Build history of the part. All positions in model axes, mm. A direction names the side the tool comes from. Round coordinates to 2 decimals unless told otherwise and drop trailing zeros. Order: outer loops, then holes, each group sorted by start corner. A loop starts at its lowest first (then second) coordinate and runs counter-clockwise, first axis right, second up. Notation, with made-up numbers: (-34.5, 56) -> (22.5, 56) arc R27 ccw to (22.5, 76) -> close; hole circle Ø3 at (-38.5, -16). An arc over 180 degrees is marked (long way). Use a Markdown table: item, result. Add a question column.
Item 1: 3-axis set-ups, long thin cutter, end or side, ignore diameter. For faces 1 (the face through (-25.126, -37, 2)), 2 (the face through (-9.126, 36, 6)), 3 (the face through (-15.126, -43, 6)): which of +Z, -Z, +X, -X, +Y, -Y reach the whole face in a straight line?
Item 2: Slice it at A-A, the plane y = -38.5. Give the cut face in (x, z), plus the area to 3 significant figures.
Item 3: Pin check, flat tips, straight feed: pin 1 (3 mm diameter, centred on y = -10.5, z = 3, fed in from -X); pin 2 (2 mm diameter, centred on y = 29.5, z = 2.5, fed in from +X); pin 3 (2.5 mm diameter, centred on x = 8.5, z = 6, fed in from +Y). Stop position of each tip, or through.
Item 4: Probe L1, parallel to X at y = -49, z = 5.25; L2, parallel to X at y = 35, z = 3; L3, parallel to Z at x = 5, y = -50. List the from-to ranges inside material, lowest first.
Item 5: Slice it at C-C, the plane z = 1.25. Give the cut face in (x, y).
Item 6: Slice it at B-B, the plane x = -3. Give the cut face in (y, z).
Item 7: Slice it at D-D, the plane x = 7. Give the cut face in (y, z).
Item 8: Two-plate mould, pull along X, no slides. Class faces 4 (the face through (10.898, -51.172, 4.493)), 5 (the face through (22, -52.203, 5)), 6 (the face through (34.02, 42.04, 1.97)): released by +X, released by -X, zero draft, split by the parting line, or undercut.
from build123d import *

# Parameters (mm, degrees)
F0_R     = 2
F1_DEPTH = 4
F2_DEPTH = 5
F3_DEPTH = 7
F4_DEPTH = 5


with BuildPart() as f1:
    # F0 (on Top) → F1 (new body)
    with BuildSketch(Plane.XY):
        with BuildLine():
            Line((-15.1260387235, -59.4521127641), (26.8739612765, -59.4521127641))
            ThreePointArc((26.8739612765, -59.4521127641), (33.9450290884, -56.523180576), (36.8739612765, -49.4521127641))
            Line((36.8739612765, -49.4521127641), (36.8739612765, -26.7764899186))
            ThreePointArc((36.8739612765, -26.7764899186), (37.7418043208, -22.7017249762), (40.1947031436, -19.3342113163))
            ThreePointArc((40.1947031436, -19.3342113163), (41.1909257037, -17.1015277356), (40.1947031436, -14.8688441549))
            ThreePointArc((40.1947031436, -14.8688441549), (38.3782162175, -12.7012518837), (37.2412258633, -10.1117859269))
            ThreePointArc((37.2412258633, -10.1117859269), (38.1325390814, -7.9403059804), (39.5054840686, -6.0364187796))
            ThreePointArc((39.5054840686, -6.0364187796), (40.4532524775, -3.6015277356), (39.5054840686, -1.1666366915))
            ThreePointArc((39.5054840686, -1.1666366915), (38.0314315628, 0.9238685756), (37.135949584, 3.3199393357))
            ThreePointArc((37.135949584, 3.3199393357), (38.0470763022, 5.745513105), (39.5508012398, 7.8555773976))
            ThreePointArc((39.5508012398, 7.8555773976), (40.3538532288, 9.8984722644), (39.5508012398, 11.9413671312))
            ThreePointArc((39.5508012398, 11.9413671312), (37.5672002834, 15.092574421), (36.8739612765, 18.7510166874))
            Line((36.8739612765, 18.7510166874), (36.8739612765, 35.0460018218))
            ThreePointArc((36.8739612765, 35.0460018218), (33.9450290884, 42.1170696336), (26.8739612765, 45.0460018218))
            Line((26.8739612765, 45.0460018218), (-15.1260387235, 45.0460018218))
            ThreePointArc((-15.1260387235, 45.0460018218), (-22.1971065353, 42.1170696336), (-25.1260387235, 35.0460018218))
            Line((-25.1260387235, 35.0460018218), (-25.1260387235, 19.9840717389))
            Line((-25.1260387235, 19.9840717389), (-25.1260387235, 18.5548229328))
            ThreePointArc((-25.1260387235, 18.5548229328), (-25.7654117274, 15.0364906233), (-27.6017711715, 11.9680636533))
            ThreePointArc((-27.6017711715, 11.9680636533), (-28.3444909059, 9.9920358694), (-27.6017711715, 8.0160080856))
            ThreePointArc((-27.6017711715, 8.0160080856), (-26.1525927882, 5.8425546017), (-25.3157639737, 3.3679363345))
            ThreePointArc((-25.3157639737, 3.3679363345), (-26.0961993133, 1.0098808841), (-27.4337310312, -1.0830868009))
            ThreePointArc((-27.4337310312, -1.0830868009), (-28.1260387235, -3), (-27.4337310312, -4.9169131991))
            ThreePointArc((-27.4337310312, -4.9169131991), (-26.0675201626, -7.0706775127), (-25.2905870197, -9.5))
            ThreePointArc((-25.2905870197, -9.5), (-26.0675201626, -11.9293224873), (-27.4337310312, -14.0830868009))
            ThreePointArc((-27.4337310312, -14.0830868009), (-28.1260387235, -16), (-27.4337310312, -17.9169131991))
            ThreePointArc((-27.4337310312, -17.9169131991), (-25.7206392922, -20.9097927605), (-25.1260387235, -24.3066238629))
            Line((-25.1260387235, -24.3066238629), (-25.1260387235, -49.4521127641))
            ThreePointArc((-25.1260387235, -49.4521127641), (-22.1971065353, -56.523180576), (-15.1260387235, -59.4521127641))
        make_face()
        with Locations((6.253258194, -49.4241423296)):
            Circle(F0_R, mode=Mode.SUBTRACT)
        with BuildLine():
            Line((-16.1260387235, 37.7969445288), (-9.1260387235, 37.7969445288))
            Line((-9.1260387235, 37.7969445288), (20.6900215282, 37.7969445288))
            Line((20.6900215282, 37.7969445288), (27.8739612765, 37.7969445288))
            ThreePointArc((27.8739612765, 37.7969445288), (29.9952816201, 36.9182648724), (30.8739612765, 34.7969445288))
            Line((30.8739612765, 34.7969445288), (30.8739612765, 27.7969445288))
            Line((30.8739612765, 27.7969445288), (30.8739612765, -42.2030554712))
            Line((30.8739612765, -42.2030554712), (30.8739612765, -49.2030554712))
            ThreePointArc((30.8739612765, -49.2030554712), (29.9952816201, -51.3243758147), (27.8739612765, -52.2030554712))
            Line((27.8739612765, -52.2030554712), (20.8739612765, -52.2030554712))
            Line((20.8739612765, -52.2030554712), (13.9387492757, -52.2030554712))
            ThreePointArc((13.9387492757, -52.2030554712), (10.9338280149, -51.199359791), (9.1353173496, -48.5912347577))
            ThreePointArc((9.1353173496, -48.5912347577), (6.253258194, -46.4241423296), (3.3711990383, -48.5912347577))
            ThreePointArc((3.3711990383, -48.5912347577), (1.572688373, -51.199359791), (-1.4322328878, -52.2030554712))
            Line((-1.4322328878, -52.2030554712), (-9.1260387235, -52.2030554712))
            Line((-9.1260387235, -52.2030554712), (-16.1260387235, -52.2030554712))
            ThreePointArc((-16.1260387235, -52.2030554712), (-18.247359067, -51.3243758147), (-19.1260387235, -49.2030554712))
            Line((-19.1260387235, -49.2030554712), (-19.1260387235, -42.2030554712))
            Line((-19.1260387235, -42.2030554712), (-19.1260387235, 27.7969445288))
            Line((-19.1260387235, 27.7969445288), (-19.1260387235, 34.7969445288))
            ThreePointArc((-19.1260387235, 34.7969445288), (-18.247359067, 36.9182648724), (-16.1260387235, 37.7969445288))
        make_face(mode=Mode.SUBTRACT)
        with BuildLine():
            ThreePointArc((36.8739612765, -7.4265655526), (36.9662028486, -8.7816754868), (37.2412258633, -10.1117859269))
            ThreePointArc((37.2412258633, -10.1117859269), (36.9662028486, -11.441896367), (36.8739612765, -12.7970063012))
            Line((36.8739612765, -12.7970063012), (36.8739612765, -7.4265655526))
        make_face(mode=Mode.SUBTRACT)
        with BuildLine():
            ThreePointArc((36.8739612765, -12.7970063012), (36.9662028486, -11.441896367), (37.2412258633, -10.1117859269))
            ThreePointArc((37.2412258633, -10.1117859269), (36.9662028486, -8.7816754868), (36.8739612765, -7.4265655526))
            Line((36.8739612765, -7.4265655526), (36.8739612765, -12.7970063012))
        make_face()
    extrude(amount=F1_DEPTH)

    # F0 (on Top) → F2 (join)
    with BuildSketch(Plane.XY):
        with BuildLine():
            Line((20.6900215282, 37.7969445288), (-9.1260387235, 37.7969445288))
            Line((-9.1260387235, 37.7969445288), (-9.1260387235, 33.7969445288))
            Line((-9.1260387235, 33.7969445288), (-10.1260387235, 33.7969445288))
            ThreePointArc((-10.1260387235, 33.7969445288), (-13.6615726294, 32.3324784348), (-15.1260387235, 28.7969445288))
            Line((-15.1260387235, 28.7969445288), (-15.1260387235, 27.7969445288))
            Line((-15.1260387235, 27.7969445288), (-19.1260387235, 27.7969445288))
            Line((-19.1260387235, 27.7969445288), (-19.1260387235, -42.2030554712))
            Line((-19.1260387235, -42.2030554712), (-15.1260387235, -42.2030554712))
            Line((-15.1260387235, -42.2030554712), (-15.1260387235, -44.2030554712))
            ThreePointArc((-15.1260387235, -44.2030554712), (-13.9544658482, -47.0314825959), (-11.1260387235, -48.2030554712))
            Line((-11.1260387235, -48.2030554712), (-9.1260387235, -48.2030554712))
            Line((-9.1260387235, -48.2030554712), (-9.1260387235, -52.2030554712))
            Line((-9.1260387235, -52.2030554712), (-1.4322328878, -52.2030554712))
            ThreePointArc((-1.4322328878, -52.2030554712), (1.572688373, -51.199359791), (3.3711990383, -48.5912347577))
            ThreePointArc((3.3711990383, -48.5912347577), (6.253258194, -46.4241423296), (9.1353173496, -48.5912347577))
            ThreePointArc((9.1353173496, -48.5912347577), (10.9338280149, -51.199359791), (13.9387492757, -52.2030554712))
            Line((13.9387492757, -52.2030554712), (20.8739612765, -52.2030554712))
            Line((20.8739612765, -52.2030554712), (20.8739612765, -48.2030554712))
            Line((20.8739612765, -48.2030554712), (22.8739612765, -48.2030554712))
            ThreePointArc((22.8739612765, -48.2030554712), (25.7023884013, -47.0314825959), (26.8739612765, -44.2030554712))
            Line((26.8739612765, -44.2030554712), (26.8739612765, -42.2030554712))
            Line((26.8739612765, -42.2030554712), (30.8739612765, -42.2030554712))
            Line((30.8739612765, -42.2030554712), (30.8739612765, 27.7969445288))
            Line((30.8739612765, 27.7969445288), (26.8739612765, 27.7969445288))
            Line((26.8739612765, 27.7969445288), (26.8739612765, 28.7969445288))
            ThreePointArc((26.8739612765, 28.7969445288), (25.4094951825, 32.3324784348), (21.8739612765, 33.7969445288))
            Line((21.8739612765, 33.7969445288), (20.6900215282, 33.7969445288))
            Line((20.6900215282, 33.7969445288), (20.6900215282, 37.7969445288))
        make_face()
    extrude(amount=F2_DEPTH)

    # F0 (on Top) → F3 (join)
    with BuildSketch(Plane.XY):
        with BuildLine():
            Line((27.8739612765, 37.7969445288), (20.6900215282, 37.7969445288))
            Line((20.6900215282, 37.7969445288), (20.6900215282, 33.7969445288))
            Line((20.6900215282, 33.7969445288), (21.8739612765, 33.7969445288))
            ThreePointArc((21.8739612765, 33.7969445288), (25.4094951825, 32.3324784348), (26.8739612765, 28.7969445288))
            Line((26.8739612765, 28.7969445288), (26.8739612765, 27.7969445288))
            Line((26.8739612765, 27.7969445288), (30.8739612765, 27.7969445288))
            Line((30.8739612765, 27.7969445288), (30.8739612765, 34.7969445288))
            ThreePointArc((30.8739612765, 34.7969445288), (29.9952816201, 36.9182648724), (27.8739612765, 37.7969445288))
        make_face()
        with BuildLine():
            Line((-9.1260387235, 33.7969445288), (-9.1260387235, 37.7969445288))
            Line((-9.1260387235, 37.7969445288), (-16.1260387235, 37.7969445288))
            ThreePointArc((-16.1260387235, 37.7969445288), (-18.247359067, 36.9182648724), (-19.1260387235, 34.7969445288))
            Line((-19.1260387235, 34.7969445288), (-19.1260387235, 27.7969445288))
            Line((-19.1260387235, 27.7969445288), (-15.1260387235, 27.7969445288))
            Line((-15.1260387235, 27.7969445288), (-15.1260387235, 28.7969445288))
            ThreePointArc((-15.1260387235, 28.7969445288), (-13.6615726294, 32.3324784348), (-10.1260387235, 33.7969445288))
            Line((-10.1260387235, 33.7969445288), (-9.1260387235, 33.7969445288))
        make_face()
        with BuildLine():
            Line((30.8739612765, -49.2030554712), (30.8739612765, -42.2030554712))
            Line((30.8739612765, -42.2030554712), (26.8739612765, -42.2030554712))
            Line((26.8739612765, -42.2030554712), (26.8739612765, -44.2030554712))
            ThreePointArc((26.8739612765, -44.2030554712), (25.7023884013, -47.0314825959), (22.8739612765, -48.2030554712))
            Line((22.8739612765, -48.2030554712), (20.8739612765, -48.2030554712))
            Line((20.8739612765, -48.2030554712), (20.8739612765, -52.2030554712))
            Line((20.8739612765, -52.2030554712), (27.8739612765, -52.2030554712))
            ThreePointArc((27.8739612765, -52.2030554712), (29.9952816201, -51.3243758147), (30.8739612765, -49.2030554712))
        make_face()
        with BuildLine():
            Line((-15.1260387235, -42.2030554712), (-19.1260387235, -42.2030554712))
            Line((-19.1260387235, -42.2030554712), (-19.1260387235, -49.2030554712))
            ThreePointArc((-19.1260387235, -49.2030554712), (-18.247359067, -51.3243758147), (-16.1260387235, -52.2030554712))
            Line((-16.1260387235, -52.2030554712), (-9.1260387235, -52.2030554712))
            Line((-9.1260387235, -52.2030554712), (-9.1260387235, -48.2030554712))
            Line((-9.1260387235, -48.2030554712), (-11.1260387235, -48.2030554712))
            ThreePointArc((-11.1260387235, -48.2030554712), (-13.9544658482, -47.0314825959), (-15.1260387235, -44.2030554712))
            Line((-15.1260387235, -44.2030554712), (-15.1260387235, -42.2030554712))
        make_face()
    extrude(amount=F3_DEPTH)

    # F0 (on Top) → F4 (join)
    with BuildSketch(Plane.XY):
        with Locations((6.253258194, -49.4241423296)):
            Circle(F0_R)
    extrude(amount=F4_DEPTH)


solid = f1.part
Check sheet entries:
| question | item | result |
|---|---|---|
| 1 | face 1 | +Z, -Z, -X, -Y |
| 1 | face 2 | +Z, +Y, -Y |
| 1 | face 3 | +Z |
| 2 | outline | (-25.13, 0) -> (36.87, 0) -> (36.87, 4) -> (30.87, 4) -> (30.87, 5) -> (-19.13, 5) -> (-19.13, 4) -> (-25.13, 4) -> close |
| 2 | area | 298 mm2 |
| 3 | pin 1 | x = -26.1 |
| 3 | pin 2 | x = 36.87 |
| 3 | pin 3 | y = 37.8 |
| 4 | L1 | -19.13 to -9.13, 20.87 to 30.87 |
| 4 | L2 | -25.13 to 36.87 |
| 4 | L3 | 0 to 5 |
| 5 | outline | (-27.6, 8.02) arc R10 cw to (-25.32, 3.37) arc R10 cw to (-27.43, -1.08) arc R3 ccw to (-27.43, -4.92) arc R10 cw to (-25.29, -9.5) arc R10 cw to (-27.43, -14.08) arc R3 ccw to (-27.43, -17.92) arc R10 cw to (-25.13, -24.31) -> (-25.13, -49.45) arc R10 ccw to (-15.13, -59.45) -> (26.87, -59.45) arc R10 ccw to (36.87, -49.45) -> (36.87, -26.78) arc R10 cw to (40.19, -19.33) arc R3 ccw to (40.19, -14.87) arc R10 cw to (37.24, -10.11) arc R10 cw to (39.51, -6.04) arc R3.6 ccw to (39.51, -1.17) arc R10 cw to (37.14, 3.32) arc R10 cw to (39.55, 7.86) arc R3 ccw to (39.55, 11.94) arc R10 cw to (36.87, 18.75) -> (36.87, 35.05) arc R10 ccw to (26.87, 45.05) -> (-15.13, 45.05) arc R10 ccw to (-25.13, 35.05) -> (-25.13, 18.55) arc R10 cw to (-27.6, 11.97) arc R3 ccw to start |
| 6 | outline | (-59.45, 0) -> (45.05, 0) -> (45.05, 4) -> (37.8, 4) -> (37.8, 5) -> (-52.2, 5) -> (-52.2, 4) -> (-59.45, 4) -> close |
| 7 | outline | (-59.45, 0) -> (45.05, 0) -> (45.05, 4) -> (37.8, 4) -> (37.8, 5) -> (-46.52, 5) -> (-46.52, 4) -> (-47.57, 4) -> (-47.57, 5) -> (-51.28, 5) -> (-51.28, 4) -> (-59.45, 4) -> close |
| 8 | face 4 | undercut |
| 8 | face 5 | zero draft |
| 8 | face 6 | released by +X |
